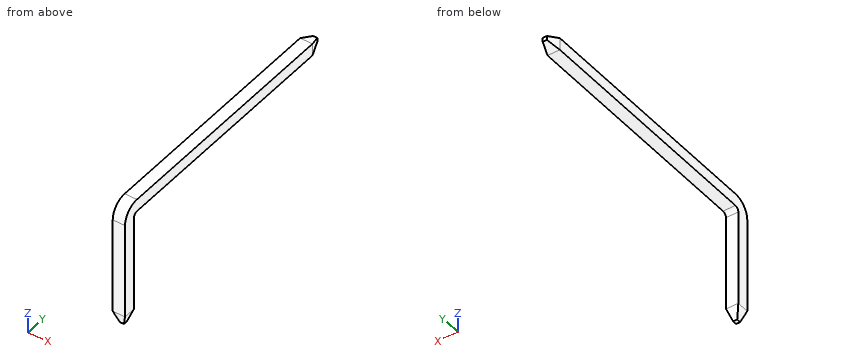
from build123d import *
from OCP.BRepFilletAPI import BRepFilletAPI_MakeChamfer

# Parameters (mm, degrees)
AUFSATZ_LINEAR_AUSTRAGEN1_DEPTH = 0.6
FASE1_SIZE                      = 0.2
FASE1_SIZE2                     = 0.6


with BuildPart() as part:
    # Skizze1 → Aufsatz-Linear austragen1 (new body)
    with BuildSketch(Plane(origin=(0, 0, 0), x_dir=(0, 0, -1), z_dir=(1, 0, 0))):
        with BuildLine():
            Line((0, 0.2), (0, 12.6))
            Line((0, 12.6), (-0.6, 12.6))
            Line((-0.6, 12.6), (-0.6, 0.2))
            ThreePointArc((-0.6, 0.2), (-0.365685425, -0.365685425), (0.2, -0.6))
            Line((0.2, -0.6), (5.5, -0.6))
            Line((5.5, -0.6), (5.5, 0))
            Line((5.5, 0), (0.2, 0))
            ThreePointArc((0.2, 0), (0.058578644, 0.058578644), (0, 0.2))
        make_face()
    extrude(amount=AUFSATZ_LINEAR_AUSTRAGEN1_DEPTH)

    # Fase1: one chamfer whose edges measure the first distance from different faces: ONE call of the kernel's chamfer builder (chamfer() names one face for all edges)
    fase1_edges_1 = [part.edges().sort_by_distance(p)[0] for p in [
        (0, 12.6, 0.3),
        (0.3, 12.6, 0),
        (0.3, 12.6, 0.6),
        (0.6, 12.6, 0.3),
    ]]
    fase1_side_1 = [part.faces().sort_by_distance(p)[0] for p in [
        (0.3, 12.6, 0.3),
    ]]
    fase1_edges_2 = [part.edges().sort_by_distance(p)[0] for p in [
        (0.3, 0, -5.5),
        (0.3, -0.6, -5.5),
        (0.6, -0.3, -5.5),
        (0, -0.3, -5.5),
    ]]
    fase1_side_2 = [part.faces().sort_by_distance(p)[0] for p in [
        (0.3, -0.3, -5.5),
    ]]
    fase1 = BRepFilletAPI_MakeChamfer(part.part.solid().wrapped)
    for e in fase1_edges_1:
        fase1.Add(FASE1_SIZE, FASE1_SIZE2, e.wrapped, fase1_side_1[0].wrapped)  # the first distance lies on this face
    for e in fase1_edges_2:
        fase1.Add(FASE1_SIZE, FASE1_SIZE2, e.wrapped, fase1_side_2[0].wrapped)  # the first distance lies on this face
    add(Compound.cast(fase1.Shape()), mode=Mode.REPLACE)


solid = part.part
Verification items for the finished model (mm, model axes). Coordinates: 2 decimals unless noted, no trailing zeros. Order: outer loops, then holes, each group sorted by start corner. A loop starts at its lowest first (then second) coordinate and runs counter-clockwise, first axis right, second up.
Item 1: Section check C-C, the plane y = 5.5. Enter the section's corners in (x, z), then the cut area to 3 significant figures.
Filled in:
outline: (0, 0) - (0.6, 0) - (0.6, 0.6) - (0, 0.6) - close
area: 0.360 mm2
Item 2: Material ranges on L1, parallel to Y at x = 0.1, z = -0.75; L2, parallel to Z at x = 0.3, y = 2.75; L3, parallel to Y at x = 0.25, z = 0.25, recorded low to high.
Filled in:
L1: y = -0.6 to 0
L2: z = 0 to 0.6
L3: y = -0.46 to 12.6
Item 3: Section check A-A, the plane x = 0.5. Enter the section's corners in (y, z), then the cut area to 3 significant figures.
Filled in:
outline: (-0.6, -4.9) - (-0.5, -5.2) - (-0.1, -5.2) - (0, -4.9) - (0, -0.2) arc R0.2 cw to (0.2, 0) - (12, 0) - (12.3, 0.1) - (12.3, 0.5) - (12, 0.6) - (0.2, 0.6) arc R0.8 ccw to (-0.6, -0.2) - close
area: 10.7 mm2
Item 4: Section check B-B, the plane z = -2. Enter the section's corners in (x, y), then the cut area to 3 significant figures.
Filled in:
outline: (0, -0.6) - (0.6, -0.6) - (0.6, 0) - (0, 0) - close
area: 0.360 mm2
